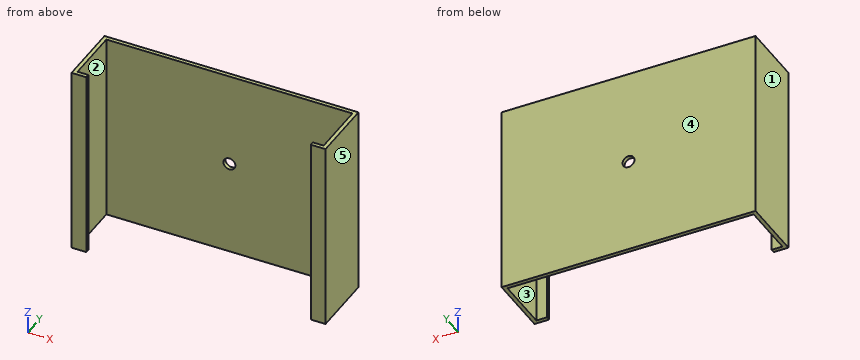
from build123d import *

# Parameters (mm, degrees)
SKETCH1_W           = 203.2
SKETCH1_H           = 50.8
SKETCH1_W_2         = 196.85
SKETCH1_H_2         = 44.45
BOSS_EXTRUDE1_DEPTH = 152.4
SKETCH2_W           = 179.578
SKETCH2_H           = 152.4
CUT_EXTRUDE1_DEPTH  = 3.175
SKETCH3_R           = 4.7625
CUT_EXTRUDE2_DEPTH  = 191.076195248


with BuildPart() as part:
    # Sketch1 → Boss-Extrude1 (new body)
    with BuildSketch(Plane.XY):
        Rectangle(SKETCH1_W, SKETCH1_H)
        Rectangle(SKETCH1_W_2, SKETCH1_H_2, mode=Mode.SUBTRACT)
    extrude(amount=BOSS_EXTRUDE1_DEPTH)

    # Sketch2 → Cut-Extrude1 (cut)
    with BuildSketch(Plane.XZ.offset(25.4)):
        with Locations((0, 76.2)):
            Rectangle(SKETCH2_W, SKETCH2_H)
    extrude(amount=-CUT_EXTRUDE1_DEPTH, mode=Mode.SUBTRACT)

    # Sketch3 → Cut-Extrude2 (cut, through all)
    with BuildSketch(Plane(origin=(0, 25.4, 0), x_dir=(1, 0, 0), z_dir=(0, 1, 0))):
        with Locations(Location((0, -76.2, 0), (0, 0, 270))):
            Circle(SKETCH3_R)
    extrude(amount=-CUT_EXTRUDE2_DEPTH, mode=Mode.SUBTRACT)


solid = part.part
Could you check a few things on this model? Use its own coordinates, in mm. Face numbers are marked on the shaded views. A direction names the side the tool comes from. Round coordinates to 2 decimals unless told otherwise and drop trailing zeros. Order: outer loops, then holes, each group sorted by start corner. A loop starts at its lowest first (then second) coordinate and runs counter-clockwise, first axis right, second up. Notation, with made-up numbers: M -23,4.5 L 7,4.5 A34 ccw 7,36.5 Z; hole C 57,72.5 d7. An arc over 180 degrees is marked long. One line per item, written item: value.
(1) Imagine slicing it at A-A (x = 0). Write out the boundary of the cut face in (y, z) (1 decimal).
Ans:
outline: M 22.2,0 L 25.4,0 L 25.4,71.4 L 22.2,71.4 Z; M 22.2,81 L 25.4,81 L 25.4,152.4 L 22.2,152.4 Z
(2) Which directions (+Z, -Z, +X, -X, +Y, -Y) give clear straight access to the entire face, cutting with the end or side of a thin tool? Please do the marked faces 1 and 2.
Ans:
face 1: +Z, -Z, -X, +Y, -Y
face 2: +Z, -Z
(3) If we mould it in two halves opening along Y, with no side actions, what happens to the marked faces 3, 4 and 5? For each: released by +Y, released by -Y, zero draft, split by the parting line, or undercut.
Ans:
face 3: undercut
face 4: released by +Y
face 5: zero draft
(4) Imagine slicing it at D-D (z = 26.5). Write out the boundary of the cut face in (x, y) (3 decimals).
Ans:
outline: M -101.6,-25.4 L -89.789,-25.4 L -89.789,-22.225 L -98.425,-22.225 L -98.425,22.225 L 98.425,22.225 L 98.425,-22.225 L 89.789,-22.225 L 89.789,-25.4 L 101.6,-25.4 L 101.6,25.4 L -101.6,25.4 Z
(5) Imagine slicing it at B-B (z = 76.2). Write out the boundary of the cut face in (x, y) (1 decimal).
Ans:
outline: M -101.6,-25.4 L -89.8,-25.4 L -89.8,-22.2 L -98.4,-22.2 L -98.4,22.2 L -4.8,22.2 L -4.8,25.4 L -101.6,25.4 Z; M 4.8,22.2 L 98.4,22.2 L 98.4,-22.2 L 89.8,-22.2 L 89.8,-25.4 L 101.6,-25.4 L 101.6,25.4 L 4.8,25.4 Z
(6) I need wall thicknesses on line 1 along X through (y, z) = (16, 26) (3 decimals); line 2 along X through (y, z) = (24.2, 76.2); line 3 along Y through (x, z) = (36.5, 109) (3 decimals). Which ranges of each line are inside material? Lowest first, please. Write a range as from..to.
Ans:
line 1: x = -101.6..-98.425, 98.425..101.6
line 2: x = -101.6..-4.76, 4.76..101.6
line 3: y = 22.225..25.4
(7) Imagine slicing it at C-C (y = -7). Write out the boundary of the cut face in (x, z) (3 decimals), and give its area (3 significant figures).
Ans:
outline: M -101.6,0 L -98.425,0 L -98.425,152.4 L -101.6,152.4 Z; M 98.425,0 L 101.6,0 L 101.6,152.4 L 98.425,152.4 Z
area: 968 mm^2
(8) I'm going to push a flat-ended pin straight in: P1, Ø2, axis at x = -62, z = 65, coming from the -Y side (3 decimals). Where does the tip first touch, or does it pass through?
Ans:
P1: stops at y = 22.225
